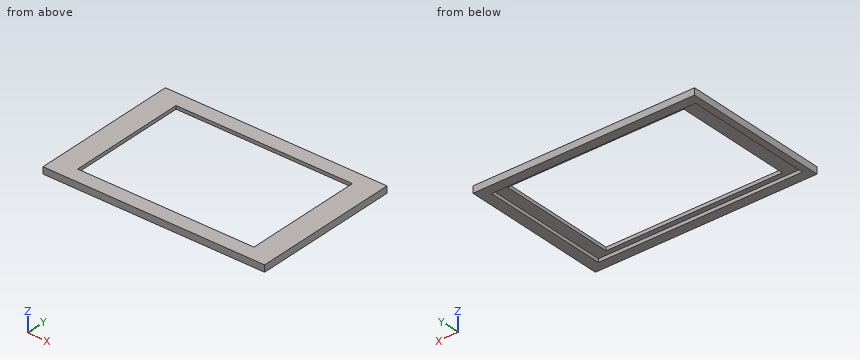
```python
from build123d import *

# Parameters (mm, degrees)
SKETCH1_W           = 113.52
SKETCH1_H           = 111.28
SKETCH1_R           = 8.5
SKETCH1_W_2         = 6
SKETCH1_H_2         = 5.8
SKETCH1_W_3         = 83.52
SKETCH1_H_3         = 56.28
BOSS_EXTRUDE1_DEPTH = 3.175
SKETCH3_W           = 96.645
SKETCH3_H           = 61.08
SKETCH3_W_2         = 83.52
SKETCH3_H_2         = 56.28
CUT_EXTRUDE1_DEPTH  = 1.5875
SKETCH4_W           = 113.52
SKETCH4_H           = 111.28
SKETCH4_W_2         = 105
SKETCH4_H_2         = 70
CUT_EXTRUDE2_DEPTH  = 10


with BuildPart() as part:
    # Sketch1 → Boss-Extrude1 (new body)
    with BuildSketch(Plane.XY):
        with Locations((0, -12.5)):
            Rectangle(SKETCH1_W, SKETCH1_H)
        with Locations((-41.76, -53.14)):
            Circle(SKETCH1_R, mode=Mode.SUBTRACT)
        with Locations((41.76, -53.14)):
            Circle(SKETCH1_R, mode=Mode.SUBTRACT)
        with Locations((-7.5, -53.14)):
            Rectangle(SKETCH1_W_2, SKETCH1_H_2, mode=Mode.SUBTRACT)
        Rectangle(SKETCH1_W_3, SKETCH1_H_3, mode=Mode.SUBTRACT)
        with Locations((-22.5, -53.14)):
            Rectangle(SKETCH1_W_2, SKETCH1_H_2, mode=Mode.SUBTRACT)
        with Locations((7.5, -53.14)):
            Rectangle(SKETCH1_W_2, SKETCH1_H_2, mode=Mode.SUBTRACT)
        with Locations((22.5, -53.14)):
            Rectangle(SKETCH1_W_2, SKETCH1_H_2, mode=Mode.SUBTRACT)
    extrude(amount=BOSS_EXTRUDE1_DEPTH)

    # Sketch3 → Cut-Extrude1 (cut)
    with BuildSketch(Plane(origin=(0, 0, 0), x_dir=(-1, 0, 0), z_dir=(0, 0, -1))):
        with Locations((0.9375, 0)):
            Rectangle(SKETCH3_W, SKETCH3_H)
        Rectangle(SKETCH3_W_2, SKETCH3_H_2, mode=Mode.SUBTRACT)
    extrude(amount=-CUT_EXTRUDE1_DEPTH, mode=Mode.SUBTRACT)

    # Sketch4 → Cut-Extrude2 (cut)
    with BuildSketch(Plane.XY.offset(3.175)):
        with Locations((0, -12.5)):
            Rectangle(SKETCH4_W, SKETCH4_H)
        Rectangle(SKETCH4_W_2, SKETCH4_H_2, mode=Mode.SUBTRACT)
    extrude(amount=-CUT_EXTRUDE2_DEPTH, mode=Mode.SUBTRACT)


solid = part.part
```
The listing builds one solid part. Answer for the finished solid, in the listing's coordinates (mm). Coordinates: 2 decimals unless noted, no trailing zeros. Write each loop counter-clockwise with the first axis right and the second up, starting at its lowest first coordinate (ties: lowest second). Pieces come first, ordered by that corner, then holes. Notation, with made-up numbers: (60.5, 26) - (117.5, 26) arc R25 ccw to (117.5, 60) - close; hole circle Ø2 at (9.25, 12.25). An arc over 180 degrees is marked (long way). Return JSON: item names as keys, results as strings. Group by question number.
Q1. Find the intervals of material crossed by line 1 along Y through (x, z) = (-5.5, 2.4); line 2 along Y through (x, z) = (41.5, 1.55); line 3 along X through (y, z) = (14, 0.85) (3 decimals), in increasing order. Write a range as [from, to].
Q2. The part is cut by section A-A on y = 0. Write down the section's boundary in (x, z) (1 decimal).
Q3. The part is cut by section C-C on x = 0. Write down the section's boundary in (y, z) (1 decimal).
Q4. The part is cut by section B-B on z = 2.1. Write down the section's boundary in (x, y).
Q5. A flat-ended cylindrical pin translates along its axis: pin 1 Ø1.5 at (x, y) = (-41.5, 18.5) entering from +Z (3 decimals). Find the tip coordinate at first contact, or state that the pin passes through.
Evaluation:
{
 "1": {"line 1": "y = [-35, -28.14], [28.14, 35]", "line 2": "y = [-35, -30.54], [30.54, 35]", "line 3": "x = [-52.5, -49.26], [47.385, 52.5]"},
 "2": {"outline": "(-52.5, 0) - (-49.3, 0) - (-49.3, 1.6) - (-41.8, 1.6) - (-41.8, 3.2) - (-52.5, 3.2) - close; (41.8, 1.6) - (47.4, 1.6) - (47.4, 0) - (52.5, 0) - (52.5, 3.2) - (41.8, 3.2) - close"},
 "3": {"outline": "(-35, 0) - (-30.5, 0) - (-30.5, 1.6) - (-28.1, 1.6) - (-28.1, 3.2) - (-35, 3.2) - close; (28.1, 1.6) - (30.5, 1.6) - (30.5, 0) - (35, 0) - (35, 3.2) - (28.1, 3.2) - close"},
 "4": {"outline": "(-52.5, -35) - (52.5, -35) - (52.5, 35) - (-52.5, 35) - close; hole (-41.76, -28.14) - (41.76, -28.14) - (41.76, 28.14) - (-41.76, 28.14) - close"},
 "5": {"pin 1": "stops at z = 3.175"}
}
